from build123d import *

# Parameters (mm, degrees)
SKETCH1_W           = 127
SKETCH1_H           = 76.2
BOSS_EXTRUDE1_DEPTH = 3.175
SKETCH2_R           = 3.25
CUT_EXTRUDE1_DEPTH  = 75.121121315


with BuildPart() as part:
    # Sketch1 → Boss-Extrude1 (new body)
    with BuildSketch(Plane(origin=(0, 0, 0), x_dir=(1, 0, 0), z_dir=(0, 1, 0))):
        Rectangle(SKETCH1_W, SKETCH1_H)
    extrude(amount=BOSS_EXTRUDE1_DEPTH)

    # Sketch2 → Cut-Extrude1 (cut, through all)
    with BuildSketch(Plane(origin=(0, 3.175, 0), x_dir=(1, 0, 0), z_dir=(0, 1, 0))):
        Polygon((63.5, -25.4), (-63.5, 12.7), (-63.5, -38.1), (63.5, -38.1), align=None)
        with Locations(Location((-53, 28.1, 0), (0, 0, 270))):
            Circle(SKETCH2_R)
        with Locations(Location((53, 28.1, 0), (0, 0, 270))):
            Circle(SKETCH2_R)
    extrude(amount=-CUT_EXTRUDE1_DEPTH, mode=Mode.SUBTRACT)


solid = part.part
Input: part model. Units: mm. Frame: model coordinates. Coordinates: 2 decimals unless noted, no trailing zeros. Write each loop counter-clockwise with the first axis right and the second up, starting at its lowest first coordinate (ties: lowest second). Pieces come first, ordered by that corner, then holes. Notation, with made-up numbers: M -26.5,15.25 L 30.5,15.25 A20 ccw 30.5,26.25 Z; hole C 31.25,83 d9. An arc over 180 degrees is marked long. Answer as a JSON object with one key per item and string values. Group by question number.
(1) Contact query for a flat-ended pin moving along its axis: P1, Ø10.5, axis at x = 53, z = -28.1, coming from the +Y side (3 decimals). Output: stop coordinate, or through.
(2) Section A-A on x = -53. Output: boundary loops of the cut face in (y, z) (3 decimals).
(3) Section B-B on z = -28.1. Output: boundary loops of the cut face in (x, y) (3 decimals), plus the area to 3 significant figures.
(4) Section D-D on x = 53. Output: boundary loops of the cut face in (y, z) (3 decimals), plus the area to 3 significant figures.
(5) Mould query, pull axis X, two halves, no side actions, for faces 1 (the face through (63.5, 2, -6)), 2 (the face through (-54.978, 1.61, -30.679)), 3 (the face through (13, 3.175, -14)). Classes: pulls with the +X half, pulls with the -X half, needs draft (parallel to the pull), parting line crosses it, or undercut.
(6) Section C-C on y = 1.1. Output: boundary loops of the cut face in (x, z).
(7) Ray query, line 1 along X through (y, z) = (1.75, -28.1); line 2 along X through (y, z) = (2.45, -27); line 3 along Z through (x, y) = (-45, 2). Return the intervals inside material, ascending. Write a range as [from, to].
Result set:
{
 "1": {"P1": "stops at y = 3.175"},
 "2": {"outline": "M 0,-38.1 L 3.175,-38.1 L 3.175,-31.35 L 0,-31.35 Z; M 0,-24.85 L 3.175,-24.85 L 3.175,-9.55 L 0,-9.55 Z"},
 "3": {"outline": "M -63.5,0 L -56.25,0 L -56.25,3.175 L -63.5,3.175 Z; M -49.75,0 L 49.75,0 L 49.75,3.175 L -49.75,3.175 Z; M 56.25,0 L 63.5,0 L 63.5,3.175 L 56.25,3.175 Z", "area": "362 mm2"},
 "4": {"outline": "M 0,-38.1 L 3.175,-38.1 L 3.175,-31.35 L 0,-31.35 Z; M 0,-24.85 L 3.175,-24.85 L 3.175,22.25 L 0,22.25 Z", "area": "171 mm2"},
 "5": {"face 1": "pulls with the +X half", "face 2": "undercut", "face 3": "needs draft"},
 "6": {"outline": "M -63.5,-38.1 L 63.5,-38.1 L 63.5,25.4 L -63.5,-12.7 Z; hole C -53,-28.1 d6.5; hole C 53,-28.1 d6.5"},
 "7": {"line 1": "x = [-63.5, -56.25], [-49.75, 49.75], [56.25, 63.5]", "line 2": "x = [-63.5, -56.06], [-49.94, 49.94], [56.06, 63.5]", "line 3": "z = [-38.1, -7.15]"}
}
